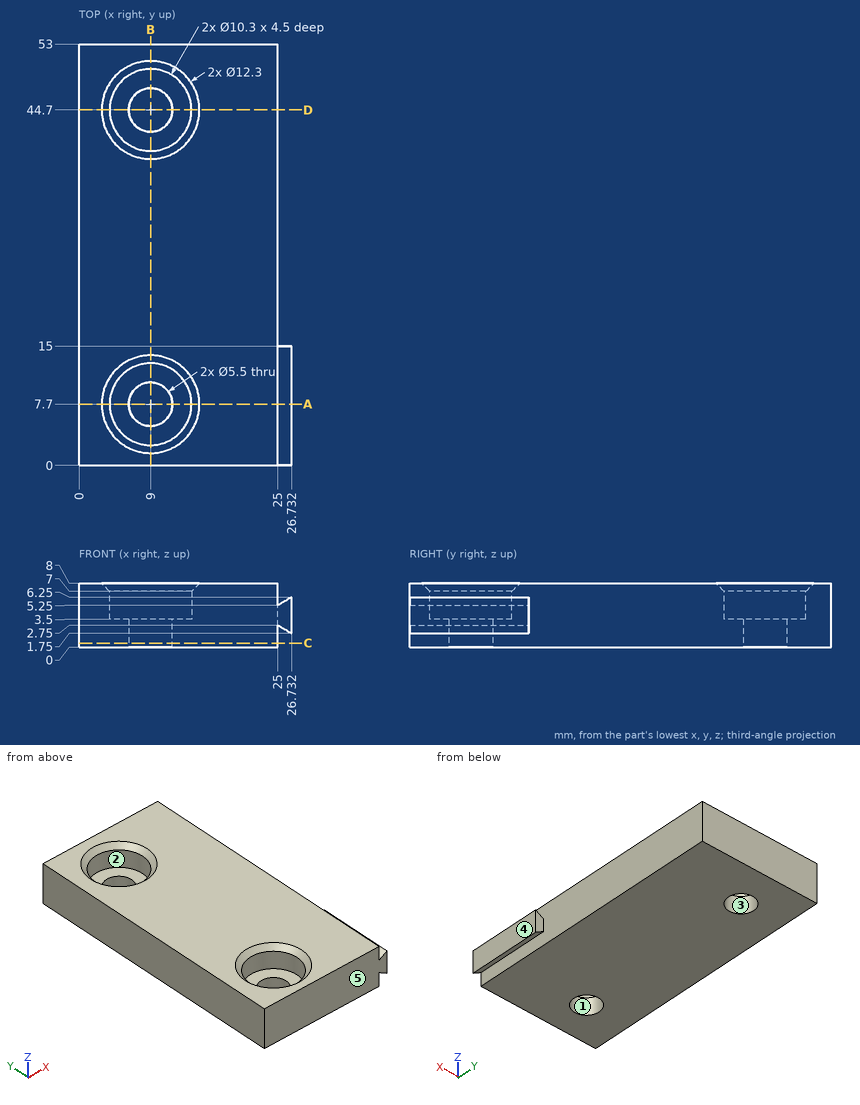
Check sheet for the drawn part. Datum: minimum x, y, z corner. Units: mm. A direction names the side the tool comes from. Give positions to 0.01 mm unless a question says otherwise; leave off trailing zeros. Write each loop counter-clockwise with the first axis right and the second up, starting at its lowest first coordinate (ties: lowest second). Pieces come first, ordered by that corner, then holes.
(1) Cross-section at D-D (y = 44.7). Enter the section's corners in (x, z), plus the area to 3 significant figures.
(2) Gauge pin test, flat ends, axial feed: pin 1 (9.5 mm diameter, centred on x = 9, y = 44.7, fed in from +Z); pin 2 (8 mm diameter, centred on x = 9.5, y = 46.5, fed in from +Z); pin 3 (0.5 mm diameter, centred on x = 26, z = 3.5, fed in from +Y). Record the tip position at first contact, or that the pin passes through.
(3) Mould release check, pull along X, two halves, no side actions. Record for the marked faces 3, 4 and 5: +X half, -X half, draft (parallel to the pull), parting line (faces both ways), or undercut.
(4) Material ranges on line 1 (Y direction, x = 9, z = 6); line 2 (Y direction, x = 9, z = 2.4); line 3 (X direction, y = 44.7, z = 2.25), recorded low to high.
(5) Access from +Z, -Z, +X, -X, +Y, -Y to the whole of each face (thin tool, end or side, straight path). Record for the marked faces 1 and 2.
(6) Cross-section at B-B (x = 9). Enter the section's corners in (y, z), plus the area to 3 significant figures.
(7) Cross-section at C-C (z = 0.5). Enter the section's corners in (x, y), plus the area to 3 significant figures.
(8) Cross-section at A-A (y = 7.7). Enter the section's corners in (x, z).
Worked out:
1. outline: (0, 0) - (6.25, 0) - (6.25, 3.5) - (3.85, 3.5) - (3.85, 7) - (2.85, 8) - (0, 8) - close; (11.75, 0) - (25, 0) - (25, 8) - (15.15, 8) - (14.15, 7) - (14.15, 3.5) - (11.75, 3.5) - close
1. area: 133 mm2
2. pin 1: stops at z = 3.5
2. pin 2: stops at z = 7.72
2. pin 3: stops at y = 15
3. face 3: undercut
3. face 4: +X half
3. face 5: draft
4. line 1: y = 0 to 2.55, 12.85 to 39.55, 49.85 to 53
4. line 2: y = 0 to 4.95, 10.45 to 41.95, 47.45 to 53
4. line 3: x = 0 to 6.25, 11.75 to 25
5. face 1: +Z, -Z
5. face 2: +Z
6. outline: (0, 0) - (4.95, 0) - (4.95, 3.5) - (2.55, 3.5) - (2.55, 7) - (1.55, 8) - (0, 8) - close; (10.45, 0) - (41.95, 0) - (41.95, 3.5) - (39.55, 3.5) - (39.55, 7) - (38.55, 8) - (13.85, 8) - (12.85, 7) - (12.85, 3.5) - (10.45, 3.5) - close; (47.45, 0) - (53, 0) - (53, 8) - (50.85, 8) - (49.85, 7) - (49.85, 3.5) - (47.45, 3.5) - close
6. area: 291 mm2
7. outline: (0, 0) - (25, 0) - (25, 53) - (0, 53) - close; hole circle Ø5.5 at (9, 7.7); hole circle Ø5.5 at (9, 44.7)
7. area: 1,280 mm2
8. outline: (0, 0) - (6.25, 0) - (6.25, 3.5) - (3.85, 3.5) - (3.85, 7) - (2.85, 8) - (0, 8) - close; (11.75, 0) - (25, 0) - (25, 2.75) - (26.73, 1.75) - (26.73, 6.25) - (25, 5.25) - (25, 8) - (15.15, 8) - (14.15, 7) - (14.15, 3.5) - (11.75, 3.5) - close
